from build123d import *

# Parameters (mm, degrees)
SKETCH1_R           = 142.5
SKETCH1_R_2         = 3.25
SKETCH1_R_3         = 37.25
SKETCH1_R_4         = 5
BOSS_EXTRUDE1_DEPTH = 25
SKETCH5_R           = 142.5
SKETCH5_R_2         = 122.5
CUT_EXTRUDE2_DEPTH  = 18


with BuildPart() as part:
    # Sketch1 → Boss-Extrude1 (new body)
    with BuildSketch(Plane.XY):
        Circle(SKETCH1_R)
        with Locations((-23.268855807, 131.964238904)):
            Circle(SKETCH1_R_2, mode=Mode.SUBTRACT)
        with Locations((23.268855807, 131.964238904)):
            Circle(SKETCH1_R_2, mode=Mode.SUBTRACT)
        with Locations((67, 116.047404107)):
            Circle(SKETCH1_R_2, mode=Mode.SUBTRACT)
        with Locations((102.649955378, 86.133539698)):
            Circle(SKETCH1_R_2, mode=Mode.SUBTRACT)
        with Locations((125.918811185, 45.830699206)):
            Circle(SKETCH1_R_2, mode=Mode.SUBTRACT)
        with Locations((134, 0)):
            Circle(SKETCH1_R_2, mode=Mode.SUBTRACT)
        with Locations((125.918811185, -45.830699206)):
            Circle(SKETCH1_R_2, mode=Mode.SUBTRACT)
        with Locations((102.649955378, -86.133539698)):
            Circle(SKETCH1_R_2, mode=Mode.SUBTRACT)
        with Locations((67, -116.047404107)):
            Circle(SKETCH1_R_2, mode=Mode.SUBTRACT)
        with Locations((23.268855807, -131.964238904)):
            Circle(SKETCH1_R_2, mode=Mode.SUBTRACT)
        with Locations((-23.268855807, -131.964238904)):
            Circle(SKETCH1_R_2, mode=Mode.SUBTRACT)
        with Locations((-67, -116.047404107)):
            Circle(SKETCH1_R_2, mode=Mode.SUBTRACT)
        with Locations((-102.649955378, -86.133539698)):
            Circle(SKETCH1_R_2, mode=Mode.SUBTRACT)
        with Locations((-125.918811185, -45.830699206)):
            Circle(SKETCH1_R_2, mode=Mode.SUBTRACT)
        with Locations((-134, 0)):
            Circle(SKETCH1_R_2, mode=Mode.SUBTRACT)
        with Locations((-125.918811185, 45.830699206)):
            Circle(SKETCH1_R_2, mode=Mode.SUBTRACT)
        with Locations((-102.649955378, 86.133539698)):
            Circle(SKETCH1_R_2, mode=Mode.SUBTRACT)
        with Locations((-67, 116.047404107)):
            Circle(SKETCH1_R_2, mode=Mode.SUBTRACT)
        Circle(SKETCH1_R_3, mode=Mode.SUBTRACT)
        with Locations((0, 55)):
            Circle(SKETCH1_R_4, mode=Mode.SUBTRACT)
        with Locations((55, 0)):
            Circle(SKETCH1_R_4, mode=Mode.SUBTRACT)
        with Locations((0, -55)):
            Circle(SKETCH1_R_4, mode=Mode.SUBTRACT)
        with Locations((-55, 0)):
            Circle(SKETCH1_R_4, mode=Mode.SUBTRACT)
    extrude(amount=BOSS_EXTRUDE1_DEPTH)

    # Sketch5 → Cut-Extrude2 (cut)
    with BuildSketch(Plane(origin=(0, 0, 0), x_dir=(-1, 0, 0), z_dir=(0, 0, -1))):
        Circle(SKETCH5_R)
        Circle(SKETCH5_R_2, mode=Mode.SUBTRACT)
    extrude(amount=-CUT_EXTRUDE2_DEPTH, mode=Mode.SUBTRACT)


solid = part.part
Build history of the part. All positions in model axes, mm. Round coordinates to 2 decimals unless told otherwise and drop trailing zeros. Write each loop counter-clockwise with the first axis right and the second up, starting at its lowest first coordinate (ties: lowest second). Pieces come first, ordered by that corner, then holes. Notation, with made-up numbers: M -10.75,44.25 L 2.25,44.25 A34 ccw 2.25,79.25 Z; hole C 15.5,11.25 d6. An arc over 180 degrees is marked long. Answer in a Markdown table with one row per item.
1. Saw through at D-D (z = 5.5). List the corners of the cut face in (x, y), and give its area (3 significant figures).
Geometry check:
| item | result |
|---|---|
| outline | C 0,0 d245; hole C -55,0 d10; hole C 0,0 d74.5; hole C 0,-55 d10; hole C 0,55 d10; hole C 55,0 d10 |
| area | 42,500 mm2 |
2. Mould opens along Y. For faces 1 (the face through (-105.028, 96.308, 21.451)), 2 (the face through (-60, 0, 12)), 3 (the face through (30, -30, 25)), 4 (the face through (-21.77, -134.85, 21.45)) say: +Y half, -Y half, draft (parallel to the pull), parting line (faces both ways), or undercut.
Geometry check:
| item | result |
|---|---|
| face 1 | parting line |
| face 2 | undercut |
| face 3 | draft |
| face 4 | undercut |
3. Flat gauge pins, fed straight in: P1, Ø6, axis at x = -65.5, z = 6.5, coming from the -Y side; P2, Ø6, axis at y = -34.5, z = 15.5, coming from the +X side; P3, Ø6, axis at x = 105, z = 13, coming from the +Y side. Where does each tip first touch, or does it go through?
Geometry check:
| item | result |
|---|---|
| P1 | y = -105.36 |
| P2 | x = 138.66 |
| P3 | y = 67.84 |
4. Saw through at C-C (y = 15). List the corners of the cut face in (x, z).
Geometry check:
| item | result |
|---|---|
| outline | M -141.71,18 L -121.58,18 L -121.58,0 L -34.1,0 L -34.1,25 L -141.71,25 Z; M 34.1,0 L 121.58,0 L 121.58,18 L 141.71,18 L 141.71,25 L 34.1,25 Z |
5. Probe L1, parallel to Y at x = 65, z = 18.5; L2, parallel to Y at x = 30, z = 6; L3, parallel to X at y = 14, z = 13. List the from-to ranges inside material, lowest first. Write a range as [from, to].
Geometry check:
| item | result |
|---|---|
| L1 | [-126.81, -118.61], [-113.49, 113.49], [118.61, 126.81] |
| L2 | [-118.77, -22.08], [22.08, 118.77] |
| L3 | [-121.7, -34.52], [34.52, 121.7] |
6. Saw through at B-B (x = 134). List the corners of the cut face in (y, z).
Geometry check:
| item | result |
|---|---|
| outline | M -48.48,18 L -3.25,18 L -3.25,25 L -48.48,25 Z; M 3.25,18 L 48.48,18 L 48.48,25 L 3.25,25 Z |
7. Saw through at A-A (x = 0). List the corners of the cut face in (y, z), and give its area (3 significant figures).
Geometry check:
| item | result |
|---|---|
| outline | M -142.5,18 L -122.5,18 L -122.5,0 L -60,0 L -60,25 L -142.5,25 Z; M -50,0 L -37.25,0 L -37.25,25 L -50,25 Z; M 37.25,0 L 50,0 L 50,25 L 37.25,25 Z; M 60,0 L 122.5,0 L 122.5,18 L 142.5,18 L 142.5,25 L 60,25 Z |
| area | 4,040 mm2 |
